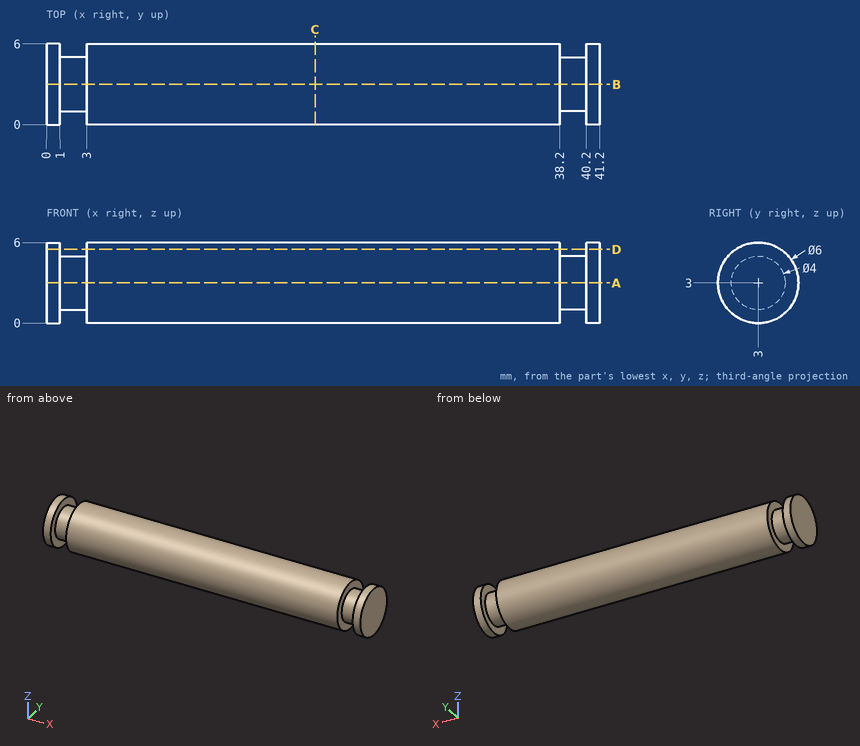
Design review of the part shown in the three views and the two pictorial views. Dimensions are in mm from the part's minimum x, y and z. Round coordinates to 2 decimals unless told otherwise and drop trailing zeros. Write each loop counter-clockwise with the first axis right and the second up, starting at its lowest first coordinate (ties: lowest second). Pieces come first, ordered by that corner, then holes.
Item 1: We need section D-D on z = 5.5. Write out the cut boundary in (x, y), and give its area (3 significant figures).
Item 2: Clearance check with a flat-ended pin moving along its axis: pin 1 Ø1.5 at (x, z) = (13.5, 1.5) entering from -Y. State where the tip first meets the part, or that it passes through.
Item 3: For probe 1 along X at (y, z) = (1.05, 4.05); probe 2 along Z at (x, y) = (35.5, 2.8); probe 3 along Y at (x, z) = (16.5, 2.3), list the stretches that pass through material, from the lowest coordinate up.
Item 4: We need section C-C on x = 20. Write out the cut boundary in (y, z), and give its area (3 significant figures).
Item 5: We need section A-A on z = 3. Write out the cut boundary in (x, y).
Returned:
1. outline: (0, 1.34) - (1, 1.34) - (1, 4.66) - (0, 4.66) - close; (3, 1.34) - (38.2, 1.34) - (38.2, 4.66) - (3, 4.66) - close; (40.2, 1.34) - (41.2, 1.34) - (41.2, 4.66) - (40.2, 4.66) - close
1. area: 123 mm2
2. pin 1: stops at y = 0.1
3. probe 1: x = 0 to 1, 3 to 38.2, 40.2 to 41.2
3. probe 2: z = 0.01 to 5.99
3. probe 3: y = 0.08 to 5.92
4. outline: circle Ø6 at (3, 3)
4. area: 28.3 mm2
5. outline: (0, 0) - (1, 0) - (1, 1) - (3, 1) - (3, 0) - (38.2, 0) - (38.2, 1) - (40.2, 1) - (40.2, 0) - (41.2, 0) - (41.2, 6) - (40.2, 6) - (40.2, 5) - (38.2, 5) - (38.2, 6) - (3, 6) - (3, 5) - (1, 5) - (1, 6) - (0, 6) - close
